from build123d import *

# Parameters (mm, degrees)
SKETCH1_W      = 40
SKETCH1_H      = 350
EXTRUDE1_DEPTH = 20
SKETCH2_R      = 7
EXTRUDE2_DEPTH = 60


with BuildPart() as part:
    # Sketch1 → Extrude1 (new body)
    with BuildSketch(Plane.XY):
        with Locations((181.317621291, 114.5)):
            Rectangle(SKETCH1_W, SKETCH1_H)
    extrude(amount=EXTRUDE1_DEPTH)

    # Sketch2 → Extrude2 (add)
    with BuildSketch(Plane(origin=(0, 0, 0), x_dir=(-1, 0, 0), z_dir=(0, 0, -1))):
        with Locations(Location((-181.317621291, -0.5, 0), (0, 0, 180))):
            Circle(SKETCH2_R)
    extrude(amount=EXTRUDE2_DEPTH)


solid = part.part
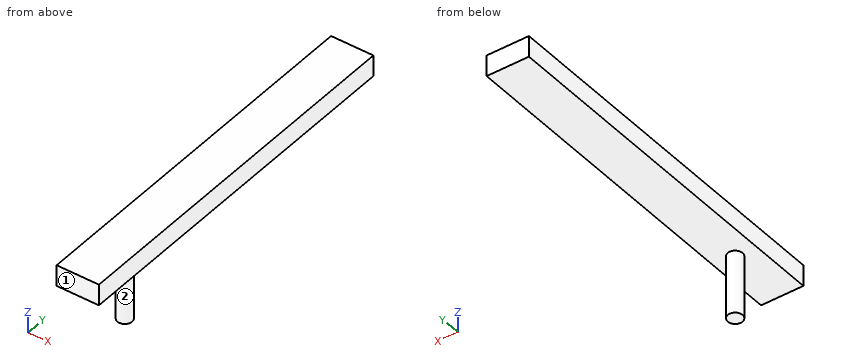
Can you work these out from the model? Positions are in its coordinate system, mm. Face numbers are marked on the shaded views. A direction names the side the tool comes from. Coordinates: 2 decimals unless noted, no trailing zeros. Order: outer loops, then holes, each group sorted by start corner. A loop starts at its lowest first (then second) coordinate and runs counter-clockwise, first axis right, second up. Notation, with made-up numbers: M 12.5,34 L 71.5,34 A20 ccw 71.5,67 Z; hole C 75,-12.5 d11. An arc over 180 degrees is marked long. Write item = value, one per line.
(1) Suppose I cut it at C-C on x = 197. Please give me the cut outline in (y, z), plus the area to 3 significant figures.
Results are:
outline = M -60.5,0 L 289.5,0 L 289.5,20 L -60.5,20 Z
area = 7,000 mm2
(2) Suppose I cut it at A-A on y = -0.5. Please give me the cut outline in (x, z).
Results are:
outline = M 161.32,0 L 174.32,0 L 174.32,-60 L 188.32,-60 L 188.32,0 L 201.32,0 L 201.32,20 L 161.32,20 Z
(3) For pin 1 Ø1.5 at (x, z) = (184, -8) entering from +Y; pin 2 Ø6 at (x, z) = (187.5, -32) entering from +Y; pin 3 Ø8 at (x, y) = (177, 252) entering from -Z, each with a flat end and sliding along its axis, tell me the tip position at first contact or that it passes through.
Results are:
pin_1 = 6.23
pin_2 = 5.73
pin_3 = 0
(4) I need wall thicknesses on line 1 along Z through (x, y) = (172.5, 164.5); line 2 along Y through (x, z) = (183, -23); line 3 along Y through (x, z) = (175.5, -34.5). Which ranges of each line are inside material? Lowest first, please. Write a range as [from, to].
Results are:
line_1 = [0, 20]
line_2 = [-7.29, 6.29]
line_3 = [-4.39, 3.39]
(5) For the marked faces 1 and 2, which set-ups out of +Z, -Z, +X, -X, +Y, -Y let a thin tool reach every point of the face, with its end or its side?
Results are:
face_1 = +Z, -Z, +X, -X, -Y
face_2 = -Z
(6) Suppose I cut it at B-B on z = -16. Please give me the cut outline in (x, y).
Results are:
outline = C 181.32,-0.5 d14
(7) Suppose I cut it at D-D on y = 225.5. Please give me the cut outline in (x, z), plus the area to 3 significant figures.
Results are:
outline = M 161.32,0 L 201.32,0 L 201.32,20 L 161.32,20 Z
area = 800 mm2
